Model file for the job. Use its own axes, mm. Face numbers are marked on the shaded views. A direction names the side the tool comes from. Coordinates: 2 decimals unless noted, no trailing zeros. Loops run counter-clockwise (first coordinate to the right, second up) from the corner with the lowest first, then second, coordinate; pieces in that order, holes last. Notation, with made-up numbers: (69.25, -13.5) -> (88.25, -13.5) arc R15 ccw to (88.25, 7.5) -> close; hole circle Ø9 at (63.25, 41). An arc over 180 degrees is marked (long way). Use one line per item in the form item = value.
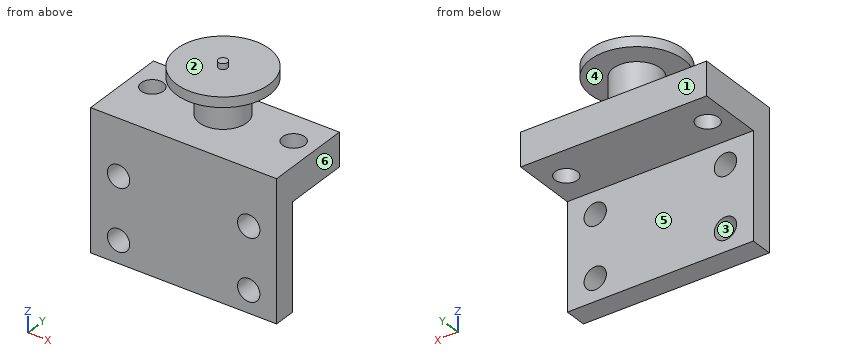
```python
from build123d import *

# Parameters (mm, degrees)
F0_W      = 100
F0_H      = 35
F1_DEPTH  = 18
F3_D      = 12
F4_R      = 12.7
F5_DEPTH  = 19
F6_R      = 25
F6_R_2    = 12.7
F7_DEPTH  = 5.5
F8_R      = 2.5
F9_DEPTH  = 3
F10_W     = 100
F10_H     = 57
F10_H_2   = 18
F11_DEPTH = 12
F13_D     = 12


with BuildPart() as f1:
    # F0 (on Top) → F1 (new body)
    with BuildSketch(Plane.XY):
        Rectangle(F0_W, F0_H)
    extrude(amount=-F1_DEPTH)

    # F3 (through all)
    with Locations(Plane.XY):
        with Locations((-38, 0), (38, 0)):
            Hole(F3_D / 2)

    # F4 (on face) → F5 (join)
    with BuildSketch(Plane.XY):
        Circle(F4_R)
    extrude(amount=F5_DEPTH)

    # F6 (on face) → F7 (join)
    with BuildSketch(Plane.XY.offset(19)):
        Circle(F6_R)
        Circle(F6_R_2, mode=Mode.SUBTRACT)
        Circle(F6_R_2)
    extrude(amount=F7_DEPTH)

    # F8 (on face) → F9 (join)
    with BuildSketch(Plane.XY.offset(24.5)):
        Circle(F8_R)
    extrude(amount=F9_DEPTH)

    # F10 (on face) → F11 (join)
    with BuildSketch(Plane.XZ.offset(17.5)):
        with Locations((0, -46.5)):
            Rectangle(F10_W, F10_H)
        with Locations((0, -9)):
            Rectangle(F10_W, F10_H_2)
    extrude(amount=F11_DEPTH)

    # F13 (through all)
    with Locations(Plane(origin=(0, -17.5, 0), x_dir=(-1, 0, 0), z_dir=(0, 1, 0))):
        with Locations((-35, -30), (-35, -63), (35, -63), (35, -30)):
            Hole(F13_D / 2)


solid = f1.part
```
Q1. Pin check, flat tips, straight feed: pin 1 Ø2 at (x, y) = (4.5, -8.5) entering from +Z; pin 2 Ø15.5 at (x, y) = (38, 0) entering from -Z; pin 3 Ø9 at (x, z) = (-17, -10.5) entering from +Y; pin 4 Ø6 at (y, z) = (-4, 1) entering from -X. Stop position of each tip, or through.
Result:
pin_1 = 24.5
pin_2 = -18
pin_3 = 17.5
pin_4 = -50
Q2. Which spindle directions (+Z, -Z, +X, -X, +Y, -Y) get a long thin tool onto all of the face, cutting with end or side? Do the marked faces 4, 5 and 6. Say none if no direction does.
Result:
face_4 = none
face_5 = -Z, +X, -X, +Y
face_6 = +Z, -Z, +X, +Y, -Y
Q3. Band-saw the part on C-C, the plane x = 0. Write the cut outline in (y, z).
Result:
outline = (-29.5, -75) -> (-17.5, -75) -> (-17.5, -18) -> (17.5, -18) -> (17.5, 0) -> (12.7, 0) -> (12.7, 19) -> (25, 19) -> (25, 24.5) -> (2.5, 24.5) -> (2.5, 27.5) -> (-2.5, 27.5) -> (-2.5, 24.5) -> (-25, 24.5) -> (-25, 19) -> (-12.7, 19) -> (-12.7, 0) -> (-29.5, 0) -> close
Q4. Band-saw the part on A-A, the plane z = -30. Write the cut outline in (x, y).
Result:
outline = (-50, -29.5) -> (-41, -29.5) -> (-41, -17.5) -> (-50, -17.5) -> close; (-29, -29.5) -> (29, -29.5) -> (29, -17.5) -> (-29, -17.5) -> close; (41, -29.5) -> (50, -29.5) -> (50, -17.5) -> (41, -17.5) -> close
Q5. Band-saw the part on D-D, the plane y = 0. Write the cut outline in (x, z), and give its area (3 significant figures).
Result:
outline = (-50, -18) -> (-44, -18) -> (-44, 0) -> (-50, 0) -> close; (-32, -18) -> (32, -18) -> (32, 0) -> (12.7, 0) -> (12.7, 19) -> (25, 19) -> (25, 24.5) -> (2.5, 24.5) -> (2.5, 27.5) -> (-2.5, 27.5) -> (-2.5, 24.5) -> (-25, 24.5) -> (-25, 19) -> (-12.7, 19) -> (-12.7, 0) -> (-32, 0) -> close; (44, -18) -> (50, -18) -> (50, 0) -> (44, 0) -> close
area = 2,140 mm2
Q6. Wall check: line 1 along Z through (x, y) = (-35, -25.5); line 2 along Z through (x, y) = (-12.5, 3); line 3 along Z through (x, y) = (-4.5, -20). Give the ranges that are in metal, low to high.
Result:
line_1 = -75 to -69, -57 to -36, -24 to 0
line_2 = -18 to 0, 19 to 24.5
line_3 = -75 to 0, 19 to 24.5
Q7. Band-saw the part on B-B, the plane y = -21. Write the cut outline in (x, z).
Result:
outline = (-50, -75) -> (50, -75) -> (50, 0) -> (-50, 0) -> close; (-13.56, 19) -> (13.56, 19) -> (13.56, 24.5) -> (-13.56, 24.5) -> close; hole circle Ø12 at (-35, -63); hole circle Ø12 at (-35, -30); hole circle Ø12 at (35, -63); hole circle Ø12 at (35, -30)
Q8. Mould opens along Z. For the marked faces 1, 2 and 3 say: released by +Z, released by -Z, zero draft, split by the parting line, or undercut.
Result:
face_1 = zero draft
face_2 = released by +Z
face_3 = undercut
